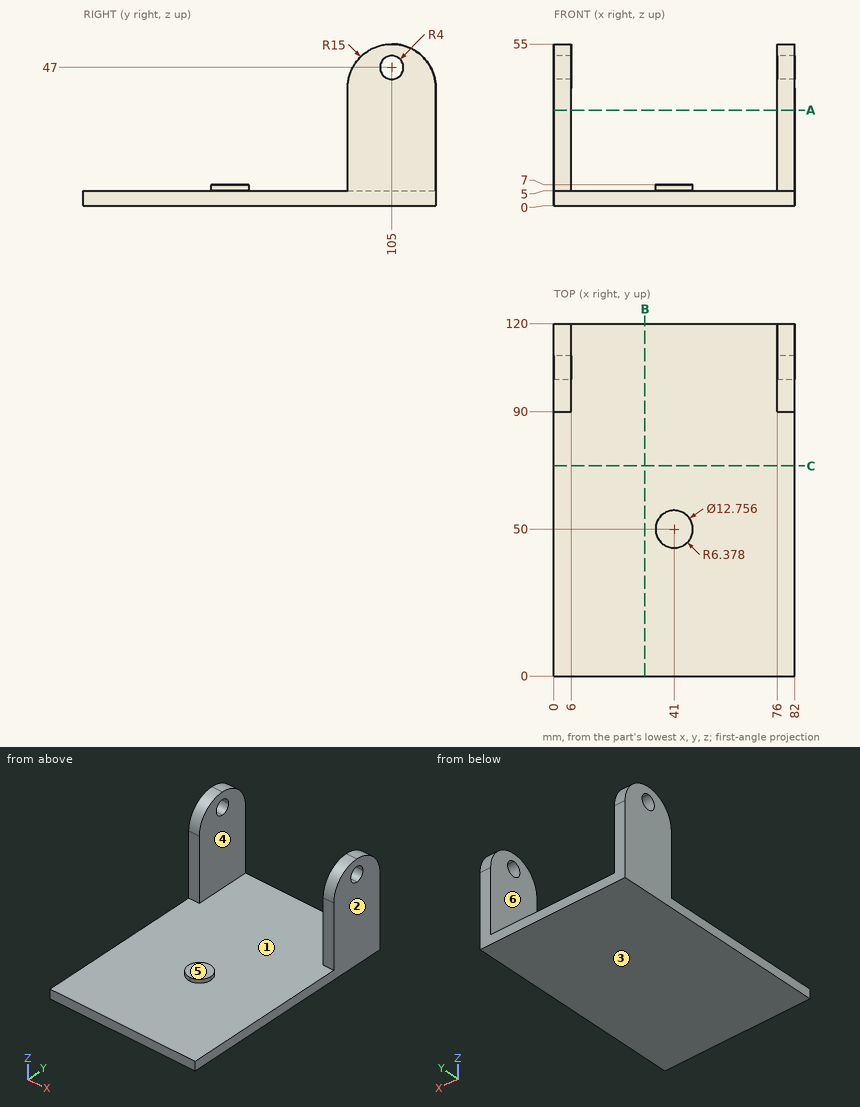
Input: dimensioned drawing with shaded views. Units: mm. Origin: part minimum x, y, z. A direction names the side the tool comes from. Coordinates: 2 decimals unless noted, no trailing zeros. Order: outer loops, then holes, each group sorted by start corner. A loop starts at its lowest first (then second) coordinate and runs counter-clockwise, first axis right, second up. Notation, with made-up numbers: (45.25, 47) - (62.25, 47) arc R22 cw to (62.25, 65) - close; hole circle Ø3 at (41, -19). An arc over 180 degrees is marked (long way). Return JSON: item names as keys, results as strings. Group by question number.
1. Cut plane A-A (z = 32.5). Output: boundary loops of the cut face in (x, y), plus the area to 3 significant figures.
2. Pull-direction query (X, two-part tool) for the marked faces 1, 2, 3 and 4; classes: pulls with the +X half, pulls with the -X half, needs draft (parallel to the pull), parting line crosses it, or undercut.
3. Cut plane C-C (y = 71.5). Output: boundary loops of the cut face in (x, z).
4. Cut plane B-B (x = 31). Output: boundary loops of the cut face in (y, z).
5. Material intervals for line 1 along X through (y, z) = (91.5, 29); line 2 along Z through (x, y) = (64.5, 94); line 3 along Y through (x, z) = (79, 36.5), sorted ascending. Write a range as [from, to].
6. Pin query (flat end, axial travel): pin 1 (12 mm diameter, centred on x = 71.5, y = 46.5, fed in from +Z); pin 2 (3 mm diameter, centred on x = 79, z = 23, fed in from -Y); pin 3 (6.5 mm diameter, centred on x = 41.5, y = 52, fed in from +Z). Return the tip coordinate at first contact, or that it passes through.
7. Set-up query: the marked faces 5 and 6. Return all of +Z, -Z, +X, -X, +Y, -Y with unobstructed straight access to the full face (end or side cutting, diameter ignored); none if empty.
Resolved:
{
 "1": {"outline": "(0, 90) - (6, 90) - (6, 120) - (0, 120) - close; (76, 90) - (82, 90) - (82, 120) - (76, 120) - close", "area": "360 mm²"},
 "2": {"face 1": "undercut", "face 2": "pulls with the +X half", "face 3": "needs draft", "face 4": "undercut"},
 "3": {"outline": "(0, 0) - (82, 0) - (82, 5) - (0, 5) - close"},
 "4": {"outline": "(0, 0) - (120, 0) - (120, 5) - (0, 5) - close"},
 "5": {"line 1": "x = [0, 6], [76, 82]", "line 2": "z = [0, 5]", "line 3": "y = [90, 120]"},
 "6": {"pin 1": "stops at z = 5", "pin 2": "stops at y = 90", "pin 3": "stops at z = 7"},
 "7": {"face 5": "+Z, +X, -X, +Y, -Y", "face 6": "+Z, +Y, -Y"}
}
